CAD build for the part. Positions are in the model's coordinates, mm. Face numbers are marked on the shaded views. A direction names the side the tool comes from. Give positions to 0.01 mm unless a question says otherwise; leave off trailing zeros. Order: outer loops, then holes, each group sorted by start corner. A loop starts at its lowest first (then second) coordinate and runs counter-clockwise, first axis right, second up. Notation, with made-up numbers: (-30, -23.5) -> (18, -23.5) arc R19 cw to (18, -7.5) -> close; hole circle Ø1 at (-28, 62.25). An arc over 180 degrees is marked (long way). Answer as CSV lines item,"result".
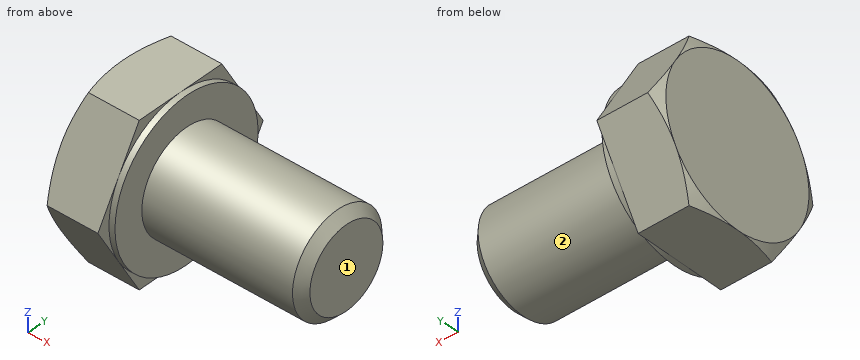
Autodesk Inventor part; units mm, degrees
ref_plane "Work Plane1" through (1.525, 0, 0) normal (0, 0, 1) x (1, 0, 0)
ref_plane "YZ Plane" through (0, 0, 0) normal (1, 0, 0) x (0, 1, 0)
ref_plane "XZ Plane" through (0, 0, 0) normal (0, 1, 0) x (-1, 0, 0)
sketch "Sketch1" plane through (0, 0, 0) normal (0, 0, 1) x (1, 0, 0)
  line L0 (0, 8) -> (0, 5)
  line L1 (4.5, 5) -> (16, 5)
  line L2 (16, 5) -> (16, 0)
  line L3 (16, 0) -> (-0.6001, 0)
  line L4 (-3.9201, 0) -> (19.32, 0)
  line L5 (-0.6001, 0) -> (-0.6001, 8)
  line L6 (-0.6001, 8) -> (0, 8)
  line L7 (4.5, 5) -> (3.5797, 5)
  line L8 (3.5797, 5) -> (0, 5)
  line L9 (0, -1.6) -> (0, 9.6)
  dimension "d0" = 16
  dimension "d1" = 11.5
  dimension "d2" = 10
  dimension "d9" = 0.6001
  dimension "d10" = 16
  dimension "d13" = 0.9203
  dimension "d14" = 10
revolve "Body" add sketch "Sketch1" angle 360 about axis through (16, 0, 0) along (-1, 0, 0)
sketch "Sketch2" plane through (-0.6001, 0, 0) normal (-1, 0, 0) x (0, 0, 1)
  line L0 (0, 9.2376) -> (8, 4.6188)
  line L1 (8, 4.6188) -> (8, -4.6188)
  line L2 (8, -4.6188) -> (0, -9.2376)
  line L3 (0, -9.2376) -> (-8, -4.6188)
  line L4 (-8, -4.6188) -> (-8, 4.6188)
  line L5 (-8, 4.6188) -> (0, 9.2376)
  point P0 (0, 0)
  point P1 (0, 0)
  dimension "d11" = 16
extrude "Head" add sketch "Sketch2" along normal blind 5.8
sketch "Sketch4" plane through (0, 0, 0) normal (0, 0, 1) x (1, 0, 0)
  line L0 (-6.4001, 8) -> (-6.4001, 9.2376)
  line L1 (-6.4001, 9.2376) -> (-5.6856, 9.2376)
  line L2 (-5.6856, 9.2376) -> (-6.4001, 8)
  line L3 (-7.5601, 0) -> (0.5599, 0)
  line L4 (-0.6001, 9.2376) -> (-6.4001, 9.2376)
  line L5 (-6.4001, 4.6188) -> (-6.4001, 9.2376)
  dimension "d5" = 30
  dimension "d19" = 16
revolve "Chamfer1" cut sketch "Sketch4" angle 360 about axis through (-10, 0, 0) along (1, 0, 0)
thread "Thread"
chamfer "Chamfer2" distance 0.9202 distance2 0.9203 1 edges at (16, -5, 0) measured on face at (16, -0.8193, 0.3214)
ref_plane "Work Plane1" through (1.525, 0, 0) normal (0, 0, 1) x (1, 0, 0)
equation "\"d11\" = SW"
equation "\"d3\" = KOH - SD"
equation "\"d15\" = GEL"
equation "\"d6\" = -0.5 * SPD + 0.5 * GD"
equation "\"d0\" = NLG"
equation "\"d1\" = GEL"
equation "\"d2\" = GD"
equation "\"d10\" = SD2"
equation "\"d14\" = BDM"
equation "\"d5\" = ANG1"
equation "\"d19\" = SW0"
equation "\"NLG\" = 16"
equation "\"GD\" = NND"
equation "\"BDM\" = NND"
equation "\"KOH\" = 6.4"
equation "\"GEL\" = 11.5"
equation "\"SW\" = 16"
equation "\"SW0\" = SW"
equation "\"SPD\" = NND - 1.2269 * PTC"
equation "\"SD2\" = SW"
equation "\"SD\" = 0.6"
equation "\"ANG1\" = 30deg"
equation "\"GAL\" = 0.61345 * PTC"
equation "\"GUL\" = 0.61345 * PTC"
equation "\"RR\" = 0.4"
equation "\"WFT\" = SD"
equation "\"GD1\" = THREADDIA - 1.2269 * PTC"
equation "\"SDH\" = SW"
equation "\"TOA\" = 30deg"
equation "\"FAWI\" = 45deg"
equation "\"PTC\" = 1.5"
equation "\"E0\" = 1.155 * SW"
properties part number "AS 1110 - M10 x 16" material "Steel, Mild"
1) Which spindle directions (+Z, -Z, +X, -X, +Y, -Y) get a long thin tool onto all of the face, cutting with end or side? Do the marked faces 1 and 2. Say none if no direction does.
Data:
face 1,"+Z, -Z, +X, +Y, -Y"
face 2,"+X"
2) Band-saw the part on B-B, the plane x = 0.75. Write the cut outline in (y, z).
Data:
outline,"circle Ø10 at (0, 0)"
3) Band-saw the part on A-A, the plane x = -2.5. Write the cut outline in (y, z), then the cut area to 3 significant figures.
Data:
outline,"(-9.24, 0) -> (-4.62, -8) -> (4.62, -8) -> (9.24, 0) -> (4.62, 8) -> (-4.62, 8) -> close"
area,"222 mm2"
4) Pin check, flat tips, straight feed: P1, Ø0.7, axis at y = -8.5, z = 0, coming from the +X side; P2, Ø3, axis at x = 11.5, z = 3.5, coming from the +Y side; P3, Ø2, axis at y = 3, z = -6, coming from the +X side. Stop position of each tip, or through.
Data:
P1,"stops at x = -0.6"
P2,"stops at y = 4.58"
P3,"stops at x = 0"
5) Wall check: line 1 along X through (y, z) = (0.25, -7); line 2 along Z through (x, y) = (2.5, 3); line 3 along Z through (x, y) = (-2.25, -7). Give the ranges that are in metal, low to high. Write a range as [from, to].
Data:
line 1,"x = [-6.4, 0]"
line 2,"z = [-4, 4]"
line 3,"z = [-3.88, 3.88]"
